from build123d import *

# Parameters (mm, degrees)
HOLE1_D           = 9.525
CIRPATTERN1_COUNT = 5


with BuildPart() as part:
    # Sketch2 → Revolve1 (revolve)
    with BuildSketch(Plane.XY):
        Polygon((-88.9, 0), (-95.25, 0), (-95.25, 57.15), (-127, 57.15), (-127, 63.5), (-101.6, 63.5), (-101.6, 88.9), (-88.9, 76.2), align=None)
    revolve(axis=Axis((0, 3.725942355, 0), (0, 1, 0)))

    # Hole1 (through all)
    with Locations(Plane(origin=(0, 63.5, 0), x_dir=(1, 0, 0), z_dir=(0, 1, 0))):
        with Locations((-114.3, 0)):
            hole1 = Hole(HOLE1_D / 2)

    # CirPattern1: Hole1 ×5 about axis
    cirpattern1_axis = Axis((0, 0, 0), (0, 1, 0))
    for i in range(1, CIRPATTERN1_COUNT):
        add(hole1.rotate(cirpattern1_axis, i * 360 / CIRPATTERN1_COUNT), mode=Mode.SUBTRACT)


solid = part.part
Design review of the part built by this model. Coordinates are the model's own, in mm. A direction names the side the tool comes from. Give positions to 0.01 mm unless a question says otherwise; leave off trailing zeros. Order: outer loops, then holes, each group sorted by start corner. A loop starts at its lowest first (then second) coordinate and runs counter-clockwise, first axis right, second up. Notation, with made-up numbers: (27.5, 88) - (61.5, 88) arc R24 ccw to (61.5, 118) - close; hole circle Ø10 at (52.25, 21.25). An arc over 180 degrees is marked (long way). Use CSV: the item, a comma, the result in double quotes. Start each with the question number.
Q1. Take a section at A-A (x = 0). State the section outline as (y, z) points, and give its area (3 significant figures).
Q2. Take a section at C-C (y = 29.5). State the section outline as (x, z) points.
Q3. Take a section at B-B (z = 0). State the section outline as (x, y) points.
Q4. Draft analysis for pull direction X (two halves, no side actions). For faces 4 (the face through (-56, 63.5, 85)), 5 (the face through (27.53, 60.37, -123.98)), 6 (the face through (95.305, 60.281, 71.011)), state which applies: pulls with the +X half, pulls with the -X half, needs draft (parallel to the pull), parting line crosses it, or undercut.
Q5. For P1, Ø8.5, axis at x = -35.32, z = 108.71, coming from the +Y side; P2, Ø10, axis at y = 42, z = 47.5, coming from the -X side; P3, Ø10, axis at y = 61, z = 89.5, coming from the +X side; P4, Ø4, axis at y = 78, z = 82, coming from the +X side, all flat-tipped, find the tip position at first contact; note any pin that passes through.
Q6. For line 1 (Y direction, x = -95.5, z = -62.5); line 2 (X direction, y = 5.5, z = 21); line 3 (X direction, y = 29.5, z = -49.5), list the stretches that pass through material, from the lowest coordinate up.
Q7. Take a section at D-D (x = -114.3). State the section outline as (y, z) points, and give its area (3 significant figures).
Q8. Machinability: for faces 1 (the face through (22.025, 76.378, -99.184)), 2 (the face through (18, 57.15, 95)), 3 (the face through (-118.843, 60.281, -1.431)), which of the approach directions +Z, -Z, +X, -X, +Y, -Y give a long, thin tool a straight path to every point of the face, cutting with its end or side? Answer none if there is none.
Calculated:
1,outline,"(0, -95.25) - (57.15, -95.25) - (57.15, -127) - (63.5, -127) - (63.5, -101.6) - (88.9, -101.6) - (76.2, -88.9) - (0, -88.9) - close; (0, 88.9) - (76.2, 88.9) - (88.9, 101.6) - (63.5, 101.6) - (63.5, 127) - (57.15, 127) - (57.15, 95.25) - (0, 95.25) - close"
1,area,"1,690 mm²"
2,outline,"circle Ø190.5 at (0, 0); hole circle Ø177.8 at (0, 0)"
3,outline,"(-127, 57.15) - (-119.06, 57.15) - (-119.06, 63.5) - (-127, 63.5) - close; (-109.54, 57.15) - (-95.25, 57.15) - (-95.25, 0) - (-88.9, 0) - (-88.9, 76.2) - (-101.6, 88.9) - (-101.6, 63.5) - (-109.54, 63.5) - close; (88.9, 0) - (95.25, 0) - (95.25, 57.15) - (127, 57.15) - (127, 63.5) - (101.6, 63.5) - (101.6, 88.9) - (88.9, 76.2) - close"
4,face 4,"needs draft"
4,face 5,"parting line crosses it"
4,face 6,"undercut"
5,P1,"passes through"
5,P2,"stops at x = -85.24"
5,P3,"stops at x = 94.81"
5,P4,"stops at x = 62.63"
6,line 1,"y = 57.15 to 63.5"
6,line 2,"x = -92.91 to -86.38, 86.38 to 92.91"
6,line 3,"x = -81.38 to -73.84, 73.84 to 81.38"
7,outline,"(57.15, -55.36) - (63.5, -55.36) - (63.5, -4.76) - (57.15, -4.76) - close; (57.15, 4.76) - (63.5, 4.76) - (63.5, 55.36) - (57.15, 55.36) - close"
7,area,"643 mm²"
8,face 1,"+Y"
8,face 2,"-Y"
8,face 3,"+Y, -Y"
